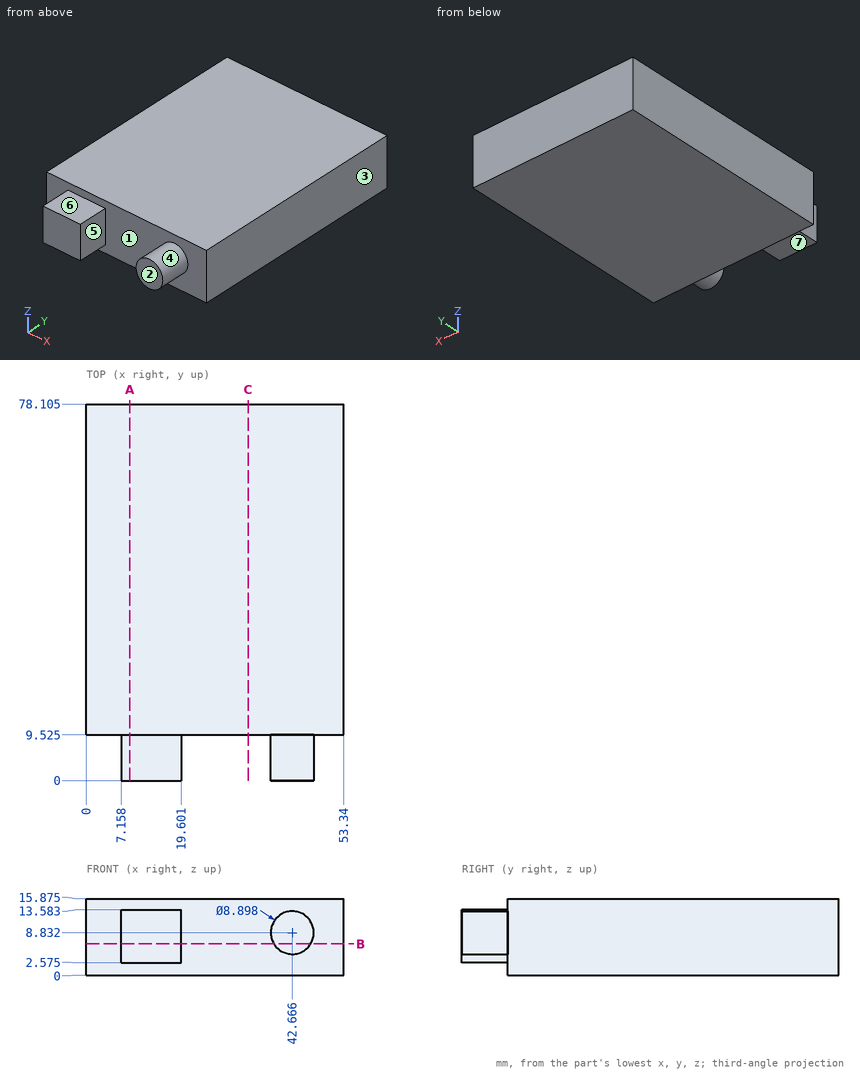
For this review, use the dimensioned drawing (mm, ordinates from the lowest corner) and the shaded views. A direction names the side the tool comes from. Coordinates: 2 decimals unless noted, no trailing zeros. Order: outer loops, then holes, each group sorted by start corner. A loop starts at its lowest first (then second) coordinate and runs counter-clockwise, first axis right, second up. Notation, with made-up numbers: (-30.75, 46.25) - (16.25, 46.25) arc R25 cw to (16.25, 76.25) - close; hole circle Ø2 at (24.5, -30). An arc over 180 degrees is marked (long way). Answer as a JSON object with one key per item and string values. Group by question number.
1. Clearance check with flat-ended pins moving along their axes: P1, Ø5, axis at y = 3, z = 7, coming from the -X side; P2, Ø4, axis at x = 24.5, z = 11.5, coming from the -Y side (3 decimals); P3, Ø5, axis at y = 2.5, z = 9.5, coming from the +X side (1 decimal). State where each tip first meets the part, or that it passes through.
2. The part is to be moulded in two halves that separate along X. For the marked faces 1, 2 and 3, say which applies: pulls with the +X half, pulls with the -X half, needs draft (parallel to the pull), parting line crosses it, or undercut.
3. We need section C-C on x = 33.5. State the section outline as (y, z) points (1 decimal).
4. We need section B-B on z = 6.5. State the section outline as (x, y) points (1 decimal), then the cut area to 3 significant figures.
5. For probe 1 along Y at (x, z) = (26.5, 12.75) (1 decimal); probe 2 along X at (y, z) = (7, 5.5) (1 decimal), list the stretches that pass through material, from the lowest coordinate up.
6. For the marked faces 4, 5, 6 and 7, list the 3-axis set-ups (+Z, -Z, +X, -X, +Y, -Y) from which the entire face can be reached by the end or side of a thin tool; tool diameter is ignored.
7. We need section A-A on x = 9. State the section outline as (y, z) points (1 decimal), then the cut area to 3 significant figures.
Final values:
{
 "1": {"P1": "x = 7.16", "P2": "y = 9.525", "P3": "x = 47.1"},
 "2": {"face 1": "undercut", "face 2": "needs draft", "face 3": "pulls with the +X half"},
 "3": {"outline": "(9.5, 0) - (78.1, 0) - (78.1, 15.9) - (9.5, 15.9) - close"},
 "4": {"outline": "(0, 9.5) - (7.2, 9.5) - (7.2, 0) - (19.6, 0) - (19.6, 9.5) - (38.9, 9.5) - (38.9, 0) - (46.5, 0) - (46.5, 9.5) - (53.3, 9.5) - (53.3, 78.1) - (0, 78.1) - close", "area": "3,850 mm²"},
 "5": {"probe 1": "9.5 to 78.1", "probe 2": "7.2 to 19.6, 39.7 to 45.6"},
 "6": {"face 4": "-Y", "face 5": "+Z, -Z, -Y", "face 6": "+Z, +X, -X, -Y", "face 7": "-Z, +X, -X, -Y"},
 "7": {"outline": "(0, 2.6) - (9.5, 2.6) - (9.5, 0) - (78.1, 0) - (78.1, 15.9) - (9.5, 15.9) - (9.5, 13.6) - (0, 13.6) - close", "area": "1,190 mm²"}
}
